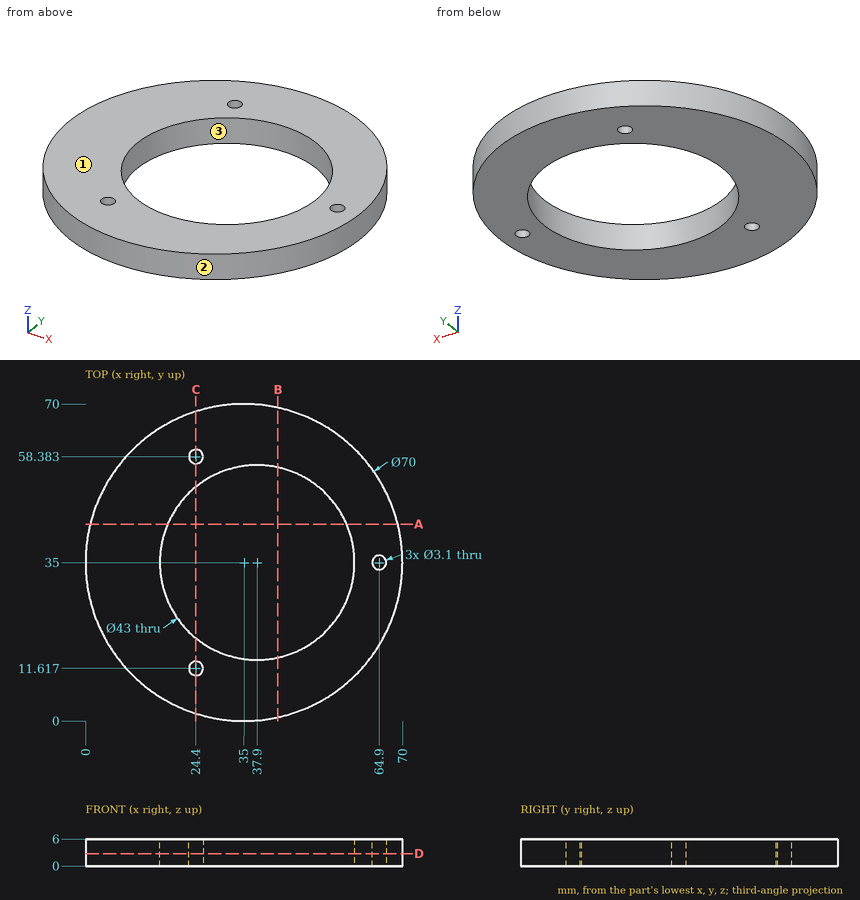
Geometry: see drawing. Coordinates: mm, zero at the bounding-box minimum. Round coordinates to 2 decimals unless told otherwise and drop trailing zeros. Loops run counter-clockwise (first coordinate to the right, second up) from the corner with the lowest first, then second, coordinate; pieces in that order, holes last. Notation, with made-up numbers: (-21.5, 14) - (25.5, 14) arc R3 ccw to (25.5, 19) - close; hole circle Ø4 at (84.5, -36.5). An arc over 180 degrees is marked (long way). One line per item, written item: value. Start each with the question number.
(1) Section B-B, the plane x = 42.5. Return loops of the section in (y, z), plus the area to 3 significant figures.
(2) Contact query for flat-ended pins moving along their axis: P1, Ø3, axis at x = 24.4, y = 58.38, coming from the -Z side; P2, Ø2, axis at x = 32.5, z = 1, coming from the +Y side; P3, Ø1.5, axis at x = 32, z = 4, coming from the -Y side. Output: stop coordinate, or through.
(3) Section A-A, the plane y = 43.5. Return loops of the section in (x, z), plus the area to 3 significant figures.
(4) Section C-C, the plane x = 24.4. Return loops of the section in (y, z).
(5) Ray query, line 1 (Y direction, x = 24, z = 1.2) (1 decimal); line 2 (Y direction, x = 24.4, z = 3.7) (1 decimal); line 3 (Y direction, x = 27.5, z = 1.85). Return the intervals inside material, ascending. Write a range as [from, to].
(6) Section D-D, the plane z = 2.75. Return loops of the section in (x, y), plus the area to 3 significant figures.
(7) Draft query along Y for the marked faces 1, 2 and 3. Return one class per face: +Y half, -Y half, draft (parallel to the pull), parting line (faces both ways), or undercut.
Results below:
1. outline: (0.81, 0) - (14, 0) - (14, 6) - (0.81, 6) - close; (56, 0) - (69.19, 0) - (69.19, 6) - (56, 6) - close
1. area: 158 mm^2
2. P1: through
2. P2: y = 69.97
2. P3: y = 0.07
3. outline: (1.05, 0) - (18.15, 0) - (18.15, 6) - (1.05, 6) - close; (57.65, 0) - (68.95, 0) - (68.95, 6) - (57.65, 6) - close
3. area: 170 mm^2
4. outline: (1.64, 0) - (10.07, 0) - (10.07, 6) - (1.64, 6) - close; (13.17, 0) - (18.27, 0) - (18.27, 6) - (13.17, 6) - close; (51.73, 0) - (56.83, 0) - (56.83, 6) - (51.73, 6) - close; (59.93, 0) - (68.36, 0) - (68.36, 6) - (59.93, 6) - close
5. line 1: [1.8, 10.1], [13.1, 18.6], [51.4, 56.9], [59.9, 68.2]
5. line 2: [1.6, 10.1], [13.2, 18.3], [51.7, 56.8], [59.9, 68.4]
5. line 3: [0.81, 16.18], [53.82, 69.19]
6. outline: circle Ø70 at (35, 35); hole circle Ø43 at (37.9, 35); hole circle Ø3.1 at (24.4, 11.62); hole circle Ø3.1 at (24.4, 58.38); hole circle Ø3.1 at (64.9, 35)
6. area: 2,370 mm^2
7. face 1: draft
7. face 2: parting line
7. face 3: undercut
